The drawing under review shows one solid part. Ordinate dimensions are in mm from its lowest x, y, z. Round coordinates to 2 decimals unless told otherwise and drop trailing zeros. Order: outer loops, then holes, each group sorted by start corner. A loop starts at its lowest first (then second) coordinate and runs counter-clockwise, first axis right, second up. Notation, with made-up numbers: M -26.5,72.25 L 29.5,72.25 A9 cw 29.5,81.25 Z; hole C -21,-20.5 d2. An arc over 180 degrees is marked long. Answer as a JSON object with one key per item and string values. Group by question number.
1. Add section C-C on y = 0.3. State the section outline as (x, z) points (3 decimals), and give its area (3 significant figures).
2. Add section B-B on z = 3.5. State the section outline as (x, y) points (1 decimal).
3. Add section D-D on z = 4.75. State the section outline as (x, y) points (3 decimals).
4. To check wall thickness, follow probe 1 along X at (y, z) = (2.5, 2); probe 2 along X at (y, z) = (1.4, 1.5) (1 decimal); probe 3 along Z at (x, y) = (7.25, 2.7). State the ranges of each line that lie inside material, in increasing order. Write a range as [from, to].
5. Clearance check with a flat-ended pin moving along its axis: P1, Ø2.5, axis at x = 5.461, z = 3.175, coming from the +Y side. State where the tip first meets the part, or that it passes through.
6. Mouldability with a two-part tool opening along Z and no side actions: class the marked faces 1, 2 and 3 as released by +Z, released by -Z, zero draft, split by the parting line, or undercut.
7. Add section A-A on x = 5. State the section outline as (y, z) points (3 decimals).
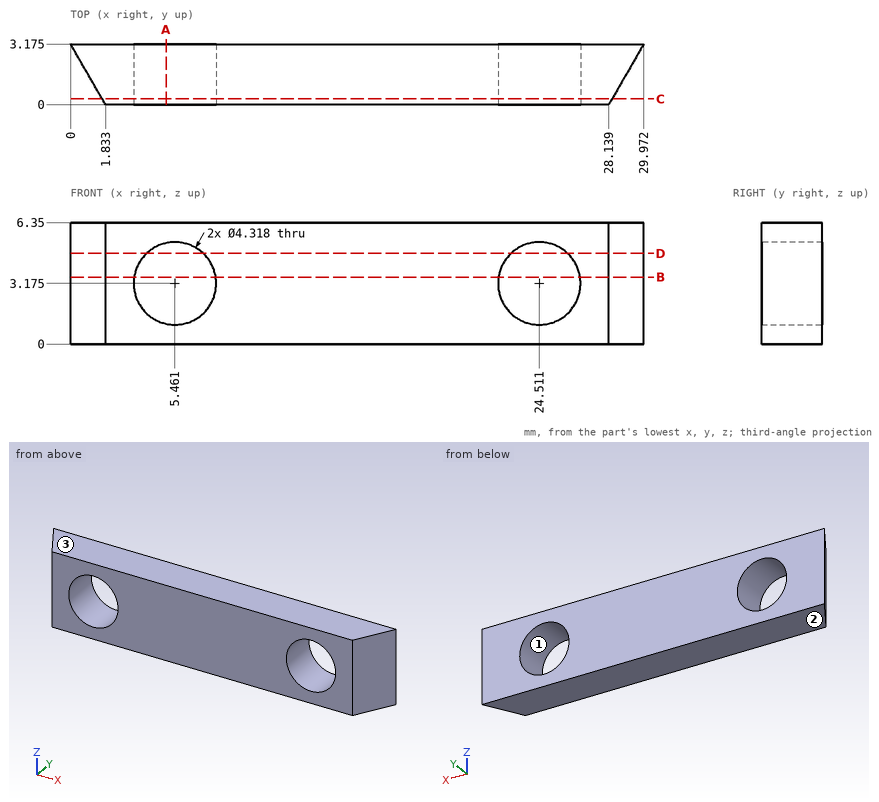
Recorded:
{
 "1": {"outline": "M 1.66,0 L 28.312,0 L 28.312,6.35 L 1.66,6.35 Z; hole C 5.461,3.175 d4.318; hole C 24.511,3.175 d4.318", "area": "140 mm²"},
 "2": {"outline": "M 0,3.2 L 1.8,0 L 3.3,0 L 3.3,3.2 Z; M 7.6,0 L 22.4,0 L 22.4,3.2 L 7.6,3.2 Z; M 26.6,0 L 28.1,0 L 30,3.2 L 26.6,3.2 Z"},
 "3": {"outline": "M 0,3.175 L 1.833,0 L 3.984,0 L 3.984,3.175 Z; M 6.938,0 L 23.034,0 L 23.034,3.175 L 6.938,3.175 Z; M 25.988,0 L 28.139,0 L 29.972,3.175 L 25.988,3.175 Z"},
 "4": {"probe 1": "x = [0.39, 3.65], [7.27, 22.7], [26.32, 29.58]", "probe 2": "x = [1, 4.1], [6.8, 23.1], [25.9, 28.9]", "probe 3": "z = [0, 1.97], [4.38, 6.35]"},
 "5": {"P1": "passes through"},
 "6": {"face 1": "undercut", "face 2": "released by -Z", "face 3": "released by +Z"},
 "7": {"outline": "M 0,0 L 3.175,0 L 3.175,1.066 L 0,1.066 Z; M 0,5.284 L 3.175,5.284 L 3.175,6.35 L 0,6.35 Z"}
}
